Can you work these out from the model? Positions are in its coordinate system, mm. Face numbers are marked on the shaded views. A direction names the side the tool comes from. Coordinates: 2 decimals unless noted, no trailing zeros. Loops run counter-clockwise (first coordinate to the right, second up) from the corner with the lowest first, then second, coordinate; pieces in that order, holes last.
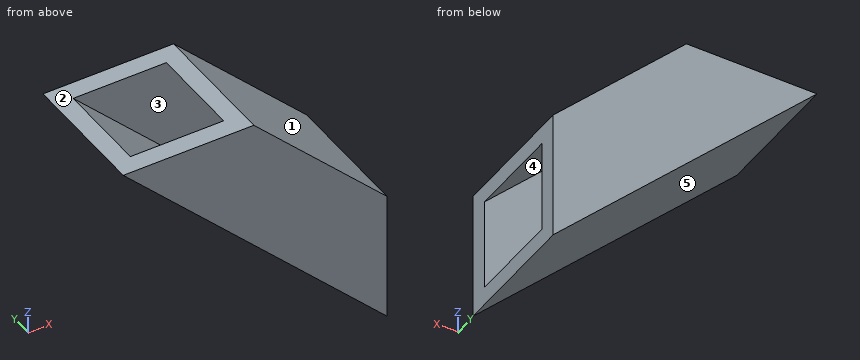
```python
from build123d import *

# Parameters (mm, degrees)
CROQUIS1_W              = 21
CROQUIS1_H              = 21
CROQUIS1_W_2            = 15
CROQUIS1_H_2            = 15
SALIENTE_EXTRUIR1_DEPTH = 70
CROQUIS6_W              = 21
CROQUIS6_H              = 21
CROQUIS6_W_2            = 15
CROQUIS6_H_2            = 15
SALIENTE_EXTRUIR2_DEPTH = 60
CORTAR_EXTRUIR2_DEPTH   = 91.234165061
CROQUIS8_W              = 21
CROQUIS8_H              = 21
CROQUIS8_W_2            = 15
CROQUIS8_H_2            = 15
SALIENTE_EXTRUIR3_DEPTH = 60
CROQUIS9_W              = 21
CROQUIS9_H              = 70
CROQUIS9_W_2            = 60
CROQUIS9_H_2            = 21
CORTAR_EXTRUIR3_DEPTH   = 118.437065189


with BuildPart() as part:
    # Croquis1 → Saliente-Extruir1 (new body)
    with BuildSketch(Plane.XY):
        Rectangle(CROQUIS1_W, CROQUIS1_H)
        Rectangle(CROQUIS1_W_2, CROQUIS1_H_2, mode=Mode.SUBTRACT)
    extrude(amount=SALIENTE_EXTRUIR1_DEPTH)

    # Croquis6 → Saliente-Extruir2 (add, along a direction that is not the sketch's normal)
    with BuildSketch(Plane(origin=(0, 0, 0), x_dir=(-1, 0, 0), z_dir=(0, 0, -1))):
        Rectangle(CROQUIS6_W, CROQUIS6_H)
        Rectangle(CROQUIS6_W_2, CROQUIS6_H_2, mode=Mode.SUBTRACT)
    extrude(amount=SALIENTE_EXTRUIR2_DEPTH, dir=(0.7071067811865512, 0, -0.7071067811865438))

    # Croquis7 → Cortar-Extruir2 (cut, through all)
    with BuildSketch(Plane(origin=(0, 10.5, 0), x_dir=(1, 0, 0), z_dir=(0, 1, 0))):
        Polygon((31.926406871, 42.426406871), (31.926406871, 21.426406871), (52.926406871, 42.426406871), align=None)
    extrude(amount=-CORTAR_EXTRUIR2_DEPTH, mode=Mode.SUBTRACT)

    # Croquis8 → Saliente-Extruir3 (add)
    with BuildSketch(Plane(origin=(31.926406871, 0, 0), x_dir=(0, 0, -1), z_dir=(1, 0, 0))):
        with Locations((31.926406871, 0)):
            Rectangle(CROQUIS8_W, CROQUIS8_H)
        with Locations((31.926406871, 0)):
            Rectangle(CROQUIS8_W_2, CROQUIS8_H_2, mode=Mode.SUBTRACT)
    extrude(amount=SALIENTE_EXTRUIR3_DEPTH)

    # Croquis9 → Cortar-Extruir3 (cut, through all)
    with BuildSketch(Plane(origin=(0, 10.5, 0), x_dir=(1, 0, 0), z_dir=(0, 1, 0))):
        with Locations((0, -35)):
            Rectangle(CROQUIS9_W, CROQUIS9_H)
        with Locations((61.926406871, 31.926406871)):
            Rectangle(CROQUIS9_W_2, CROQUIS9_H_2)
    extrude(amount=-CORTAR_EXTRUIR3_DEPTH, mode=Mode.SUBTRACT)


solid = part.part
```
Item 1: I need wall thicknesses on line 1 along Y through (x, z) = (17.5, -23); line 2 along Z through (x, y) = (27, -6.75); line 3 along X through (y, z) = (1, -4.5). Which ranges of each line are inside material? Lowest first, please.
Results are:
line 1: y = -10.5 to -7.5, 7.5 to 10.5
line 2: z = -37.5 to -34.5, -19.5 to -16.5
line 3: x = -6 to -3, 12 to 15
Item 2: I'm going to push flat-ended pins straight in: P1, Ø4, axis at y = -4, z = -20, coming from the -X side; P2, Ø2, axis at x = 7, y = -2.5, coming from the -Z side; P3, Ø5, axis at x = 14, y = 6, coming from the -Z side; P4, Ø12, axis at x = -5.5, y = -7, coming from the +Z side. Where does each tip first touch, or does it pass through?
Results are:
P1: stops at x = 7.5
P2: stops at z = -18.5
P3: stops at z = -27
P4: stops at z = 0
Item 3: Suppose I cut it at A-A, the plane y = -3.25. Please give me the cut outline in (x, z).
Results are:
outline: (-10.5, 0) - (31.93, -42.43) - (31.93, -39.43) - (-7.5, 0) - close; (7.5, 0) - (31.93, -24.43) - (31.93, -21.43) - (10.5, 0) - close
Item 4: We'd pull the mould along X, two halves only. Please class the marked faces 1, 2 and 3: +X half, -X half, draft (parallel to the pull), parting line (faces both ways), or undercut.
Results are:
face 1: +X half
face 2: draft
face 3: undercut
Item 5: Suppose I cut it at B-B, the plane z = -22. Please give me the cut outline in (x, y), plus the area to 3 significant figures.
Results are:
outline: (11.5, -10.5) - (31.93, -10.5) - (31.93, 10.5) - (11.5, 10.5) - close; hole (14.5, -7.5) - (29.5, -7.5) - (29.5, 7.5) - (14.5, 7.5) - close
area: 204 mm2
Item 6: Suppose I cut it at D-D, the plane x = -3. Please give me the cut outline in (y, z).
Results are:
outline: (-10.5, -7.5) - (10.5, -7.5) - (10.5, 0) - (7.5, 0) - (7.5, -4.5) - (-7.5, -4.5) - (-7.5, 0) - (-10.5, 0) - close
Item 7: Suppose I cut it at C-C, the plane x = 21.5. Please give me the cut outline in (y, z), plus the area to 3 significant figures.
Results are:
outline: (-10.5, -32) - (10.5, -32) - (10.5, -11) - (-10.5, -11) - close; hole (-7.5, -29) - (7.5, -29) - (7.5, -14) - (-7.5, -14) - close
area: 216 mm2
Item 8: On a 3-axis mill with a long thin cutter (end or side, diameter ignored), from which of +Z, -Z, +X, -X, +Y, -Y can I reach the whole of each face in a straight line? I mean the marked faces 4 and 5. Say none if no direction works.
Results are:
face 4: none
face 5: -Z, -X, +Y, -Y
